```python
from build123d import *

# Parameters (mm, degrees)
F0_R     = 3.81
F1_DEPTH = 3.048
F2_DEPTH = 3.048


with BuildPart() as f1:
    # F0 (on Top) → F1 (new body)
    with BuildSketch(Plane.XY):
        with BuildLine():
            ThreePointArc((5.08, 0), (-3.5921024484, -3.5921024484), (0, 5.08))
            Line((0, 5.08), (0, 10.795))
            ThreePointArc((0, 10.795), (-8.0990763391, 7.1370153042), (-10.7092601728, -1.3578554974))
            ThreePointArc((-10.7092601728, -1.3578554974), (-6.8470170962, -8.3456804327), (0.760755928, -10.7681602615))
            ThreePointArc((0.760755928, -10.7681602615), (7.8976067654, -7.3593364088), (10.795, 0))
            Line((10.795, 0), (5.08, 0))
        make_face()
        with BuildLine():
            ThreePointArc((-10.7092601728, -1.3578554974), (-8.0990763391, 7.1370153042), (0, 10.795))
            Line((0, 10.795), (0, 44.45))
            ThreePointArc((0, 44.45), (-11.3525779785, 48.2022396005), (-18.2329677514, 57.9808164576))
            Line((-18.2329677514, 57.9808164576), (-10.7092601728, -1.3578554974))
        make_face()
        with BuildLine():
            Line((0, 44.45), (0, 10.795))
            ThreePointArc((0, 10.795), (7.6332177029, 7.6332177029), (10.795, 0))
            Line((10.795, 0), (32.8899903893, 0))
            ThreePointArc((32.8899903893, 0), (35.2148303137, 5.6126600757), (40.8274903893, 7.9375))
            Line((40.8274903893, 7.9375), (20.335469936, 9.3717284546))
            ThreePointArc((20.335469936, 9.3717284546), (14.7711479184, 12.2272266722), (12.9938829963, 18.2236321774))
            Line((12.9938829963, 18.2236321774), (17.3601908133, 55.65613138))
            ThreePointArc((17.3601908133, 55.65613138), (10.3314278488, 47.4948727401), (0, 44.45))
        make_face()
        with BuildLine():
            Line((32.8899903893, 0), (10.795, 0))
            ThreePointArc((10.795, 0), (7.8976067654, -7.3593364088), (0.760755928, -10.7681602615))
            Line((0.760755928, -10.7681602615), (40.8274903893, -7.9375))
            ThreePointArc((40.8274903893, -7.9375), (35.2148303137, -5.6126600757), (32.8899903893, 0))
        make_face()
        with BuildLine():
            ThreePointArc((-18.2329677514, 57.9808164576), (-11.3525779785, 48.2022396005), (0, 44.45))
            Line((0, 44.45), (0, 59.69))
            ThreePointArc((0, 59.69), (-3.81, 63.5), (0, 67.31))
            Line((0, 67.31), (0, 82.55))
            ThreePointArc((0, 82.55), (-12.1161952262, 78.2003507863), (-18.6994561701, 67.1376969281))
            ThreePointArc((-18.6994561701, 67.1376969281), (-18.9199487116, 65.7221702793), (-19.0334427381, 64.2940765289))
            Line((-19.0334427381, 64.2940765289), (-18.2329677514, 57.9808164576))
        make_face()
        with BuildLine():
            Line((0, 59.69), (0, 44.45))
            ThreePointArc((0, 44.45), (10.3314278488, 47.4948727401), (17.3601908133, 55.65613138))
            Line((17.3601908133, 55.65613138), (18.6994561701, 67.1376969281))
            ThreePointArc((18.6994561701, 67.1376969281), (12.1161952262, 78.2003507863), (0, 82.55))
            Line((0, 82.55), (0, 67.31))
            ThreePointArc((0, 67.31), (2.6940768363, 66.1940768363), (3.81, 63.5))
            ThreePointArc((3.81, 63.5), (2.6940768363, 60.8059231637), (0, 59.69))
        make_face()
        with BuildLine():
            ThreePointArc((40.8274903893, 7.9375), (35.2148303137, 5.6126600757), (32.8899903893, 0))
            ThreePointArc((32.8899903893, 0), (35.2148303137, -5.6126600757), (40.8274903893, -7.9375))
            ThreePointArc((40.8274903893, -7.9375), (46.440150465, -5.6126600757), (48.7649903893, 0))
            ThreePointArc((48.7649903893, 0), (46.440150465, 5.6126600757), (40.8274903893, 7.9375))
        make_face()
        with BuildLine():
            ThreePointArc((45.2724903893, 0), (40.8274903893, -4.445), (36.3824903893, 0))
            ThreePointArc((36.3824903893, 0), (40.8274903893, 4.445), (45.2724903893, 0))
        make_face(mode=Mode.SUBTRACT)
        with BuildLine():
            ThreePointArc((-19.0334427381, 64.2940765289), (-18.8986944225, 61.1037844163), (-18.2329677514, 57.9808164576))
            Line((-18.2329677514, 57.9808164576), (-19.0334427381, 64.2940765289))
        make_face()
        with BuildLine():
            Line((18.6994561701, 67.1376969281), (17.3601908133, 55.65613138))
            ThreePointArc((17.3601908133, 55.65613138), (18.6227567104, 59.488088672), (19.05, 63.5))
            ThreePointArc((19.05, 63.5), (18.9621615334, 65.3272739202), (18.6994561701, 67.1376969281))
        make_face()
        with BuildLine():
            ThreePointArc((0, 82.55), (12.1161952262, 78.2003507863), (18.6994561701, 67.1376969281))
            Line((18.6994561701, 67.1376969281), (9.5247420262, 114.3))
            ThreePointArc((9.5247420262, 114.3), (9.5249355063, 114.2649490813), (9.525, 114.2298976878))
            ThreePointArc((9.525, 114.2298976878), (6.7351920908, 107.494705597), (0, 104.7048976878))
            Line((0, 104.7048976878), (0, 100.0252))
            Line((0, 100.0252), (0, 82.55))
        make_face()
        with BuildLine():
            ThreePointArc((-18.6994561701, 67.1376969281), (-12.1161952262, 78.2003507863), (0, 82.55))
            Line((0, 82.55), (0, 100.0252))
            Line((0, 100.0252), (0, 104.7048976878))
            ThreePointArc((0, 104.7048976878), (-6.7599315649, 107.5195362789), (-9.5247420262, 114.3))
            Line((-9.5247420262, 114.3), (-18.6994561701, 67.1376969281))
        make_face()
        with Locations((-3.81, 100.0252)):
            Circle(F0_R, mode=Mode.SUBTRACT)
        with BuildLine():
            ThreePointArc((9.525, 114.2298976878), (9.5249355063, 114.2649490813), (9.5247420262, 114.3))
            ThreePointArc((9.5247420262, 114.3), (0, 123.7548976878), (-9.5247420262, 114.3))
            ThreePointArc((-9.5247420262, 114.3), (-6.7599315649, 107.5195362789), (0, 104.7048976878))
            ThreePointArc((0, 104.7048976878), (6.7351920908, 107.494705597), (9.525, 114.2298976878))
        make_face()
        with BuildLine():
            ThreePointArc((3.175, 114.3), (2.2450640303, 112.0549359697), (0, 111.125))
            ThreePointArc((0, 111.125), (-2.2450640303, 116.5450640303), (3.175, 114.3))
        make_face(mode=Mode.SUBTRACT)
    extrude(amount=F1_DEPTH)

    # F0 (on Top) → F2 (join)
    with BuildSketch(Plane.XY):
        with BuildLine():
            Line((0, 10.795), (0, 5.08))
            ThreePointArc((0, 5.08), (3.5921024484, 3.5921024484), (5.08, 0))
            Line((5.08, 0), (10.795, 0))
            ThreePointArc((10.795, 0), (7.6332177029, 7.6332177029), (0, 10.795))
        make_face()
    extrude(amount=F2_DEPTH)


solid = f1.part
```
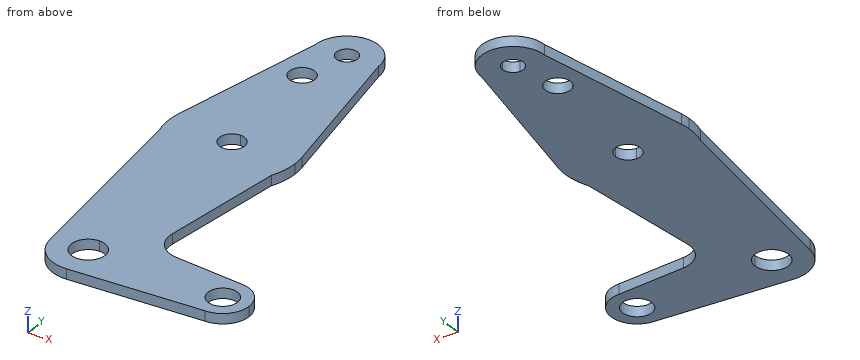
The listing builds one solid part. Answer for the finished solid, in the listing's coordinates (mm). Coordinates: 2 decimals unless noted, no trailing zeros. Write each loop counter-clockwise with the first axis right and the second up, starting at its lowest first coordinate (ties: lowest second). Pieces come first, ordered by that corner, then holes. Notation, with made-up numbers: (54.25, 27) - (78.25, 27) arc R16 cw to (78.25, 58) - close; hole circle Ø5 at (47.5, 89). An arc over 180 degrees is marked (long way). Return JSON: item names as keys, results as strings. Group by question number.
1. A cutting plane is placed at A-A, the plane z = 1.15. Give the number of separate pieces and of enclosed holes in the cut face, plus the area to 3 significant figures.
2. Straight lines are drawn through the part: L1, parallel to Y at x = 43.5, z = 1.8; L2, parallel to X at y = 66.5, z = 2.5; L3, parallel to Y at x = 4.5, z = 1.35. For each, find the intervals that lie inside material, in ascending order.
3. A cutting plane is placed at B-B, the plane y = 49. Determine the outline of the cut face in (x, z).
4. A cutting plane is placed at C-C, the plane x = 29. Determine the outline of the cut face in (y, z), plus the area to 3 significant figures.
Ans:
{
 "1": {"separate pieces": "1", "enclosed holes": "5", "area": "4,070 mm²"},
 "2": {"L1": "-7.47 to -3.55, 3.55 to 7.47", "L2": "-18.81 to -2.35, 2.35 to 18.81", "L3": "-10.5 to -2.36, 2.36 to 122.62"},
 "3": {"outline": "(-17.09, 0) - (16.58, 0) - (16.58, 3.05) - (-17.09, 3.05) - close"},
 "4": {"outline": "(-8.77, 0) - (8.77, 0) - (8.77, 3.05) - (-8.77, 3.05) - close", "area": "53.5 mm²"}
}
